from build123d import *

# Parameters (mm, degrees)
SKETCH_1_W          = 161
SKETCH_1_H          = 120
EXTRUDE_1_DEPTH     = 10
FILLET_1_R          = 10
SKETCH_2_W          = 49.5
SKETCH_2_H          = 41
CUT_EXTRUDE_1_DEPTH = 10
SKETCH_3_R          = 8.5
CUT_EXTRUDE_2_DEPTH = 10
FILLET_2_R          = 10
SKETCH_5_R          = 3.4
CUT_EXTRUDE_4_DEPTH = 118.474465311
SKETCH_6_R          = 2.6
CUT_EXTRUDE_5_DEPTH = 10


with BuildPart() as part:
    # 草图1 → 凸台-拉伸1 (new body)
    with BuildSketch(Plane(origin=(0, 0, 0), x_dir=(1, 0, 0), z_dir=(0, 1, 0))):
        with Locations((-20, 0)):
            Rectangle(SKETCH_1_W, SKETCH_1_H)
    extrude(amount=EXTRUDE_1_DEPTH)

    # 圆角1
    fillet_1_edges = [part.edges().sort_by_distance(p)[0] for p in [
        (60.5, 5, 60),
        (60.5, 5, -60),
    ]]
    fillet(fillet_1_edges, radius=FILLET_1_R)

    # 草图2 → 切除-拉伸1 (cut)
    with BuildSketch(Plane(origin=(0, 10, 0), x_dir=(1, 0, 0), z_dir=(0, 1, 0))):
        with Locations((-36.75, 0.5)):
            Rectangle(SKETCH_2_W, SKETCH_2_H)
    extrude(amount=-CUT_EXTRUDE_1_DEPTH, mode=Mode.SUBTRACT)

    # 草图3 → 切除-拉伸2 (cut)
    with BuildSketch(Plane(origin=(0, 10, 0), x_dir=(1, 0, 0), z_dir=(0, 1, 0))):
        with Locations(Location((38.5, 0, 0), (0, 0, 270))):
            Circle(SKETCH_3_R)
    extrude(amount=-CUT_EXTRUDE_2_DEPTH, mode=Mode.SUBTRACT)

    # 圆角2
    fillet_2_edges = [part.edges().sort_by_distance(p)[0] for p in [
        (-100.5, 5, 60),
        (-100.5, 5, -60),
    ]]
    fillet(fillet_2_edges, radius=FILLET_2_R)

    # 草图5 → 切除-拉伸4 (cut, through all)
    with BuildSketch(Plane.XZ):
        with Locations(Location((-40.5, 45, 0), (0, 0, 270))):
            Circle(SKETCH_5_R)
        with Locations(Location((-85.5, 0, 0), (0, 0, 270))):
            Circle(SKETCH_5_R)
        with Locations(Location((-40.5, -45, 0), (0, 0, 270))):
            Circle(SKETCH_5_R)
    extrude(amount=-CUT_EXTRUDE_4_DEPTH, mode=Mode.SUBTRACT)

    # 草图6 → 切除-拉伸5 (cut)
    with BuildSketch(Plane(origin=(0, 10, 0), x_dir=(1, 0, 0), z_dir=(0, 1, 0))):
        with Locations(Location((38.5, 24, 0), (0, 0, 270))):
            Circle(SKETCH_6_R)
        with Locations(Location((38.5, -24, 0), (0, 0, 270))):
            Circle(SKETCH_6_R)
    extrude(amount=-CUT_EXTRUDE_5_DEPTH, mode=Mode.SUBTRACT)


solid = part.part
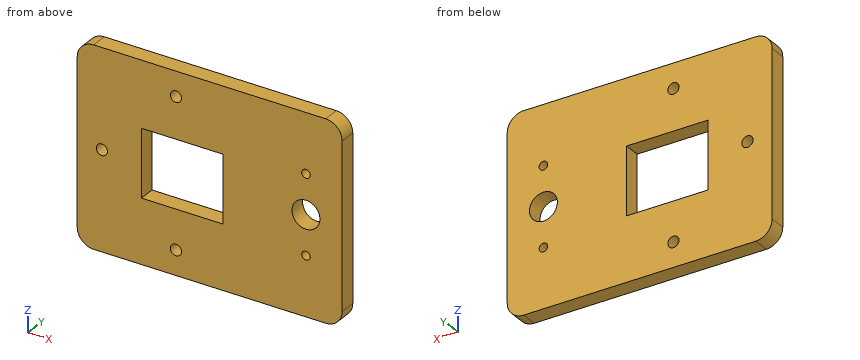
Verification items for the finished model (mm, model axes). Coordinates: 2 decimals unless noted, no trailing zeros. Loops run counter-clockwise (first coordinate to the right, second up) from the corner with the lowest first, then second, coordinate; pieces in that order, holes last. Notation, with made-up numbers: (10, -12) -> (42, -12) arc R22 cw to (42, 10) -> close; hole circle Ø10 at (-16.5, 83.25). An arc over 180 degrees is marked (long way). Answer as CSV lines item,"result".
1) Cross-section at A-A, the plane z = -24. Record the cut outline in (x, y), then the cut area to 3 significant figures.
Found:
outline,"(-100.5, 0) -> (35.9, 0) -> (35.9, 10) -> (-100.5, 10) -> close; (41.1, 0) -> (60.5, 0) -> (60.5, 10) -> (41.1, 10) -> close"
area,"1,560 mm2"
2) Cross-section at D-D, the plane z = 0. Record the cut outline in (x, y).
Found:
outline,"(-100.5, 0) -> (-88.9, 0) -> (-88.9, 10) -> (-100.5, 10) -> close; (-82.1, 0) -> (-61.5, 0) -> (-61.5, 10) -> (-82.1, 10) -> close; (-12, 0) -> (30, 0) -> (30, 10) -> (-12, 10) -> close; (47, 0) -> (60.5, 0) -> (60.5, 10) -> (47, 10) -> close"
3) Thickness scan on L1, parallel to X at y = 8, z = -2.5; L2, parallel to X at y = 4.25, z = 45; L3, parallel to X at y = 4, z = 24. Record the ranges inside material, lowest first. Write a range as from..to.
Found:
L1,"x = -100.5..-87.8, -83.2..-61.5, -12..30.38, 46.62..60.5"
L2,"x = -100.5..-43.9, -37.1..60.5"
L3,"x = -100.5..35.9, 41.1..60.5"
4) Cross-section at C-C, the plane y = 2.5. Record the cut outline in (x, z), then the cut area to 3 significant figures.
Found:
outline,"(-100.5, -50) arc R10 ccw to (-90.5, -60) -> (50.5, -60) arc R10 ccw to (60.5, -50) -> (60.5, 50) arc R10 ccw to (50.5, 60) -> (-90.5, 60) arc R10 ccw to (-100.5, 50) -> close; hole circle Ø6.8 at (-85.5, 0); hole (-61.5, -21) -> (-12, -21) -> (-12, 20) -> (-61.5, 20) -> close; hole circle Ø6.8 at (-40.5, -45); hole circle Ø6.8 at (-40.5, 45); hole circle Ø17 at (38.5, 0); hole circle Ø5.2 at (38.5, -24); hole circle Ø5.2 at (38.5, 24)"
area,"16,800 mm2"
5) Cross-section at B-B, the plane x = 38.5. Record the cut outline in (y, z).
Found:
outline,"(0, -60) -> (10, -60) -> (10, -26.6) -> (0, -26.6) -> close; (0, -21.4) -> (10, -21.4) -> (10, -8.5) -> (0, -8.5) -> close; (0, 8.5) -> (10, 8.5) -> (10, 21.4) -> (0, 21.4) -> close; (0, 26.6) -> (10, 26.6) -> (10, 60) -> (0, 60) -> close"
